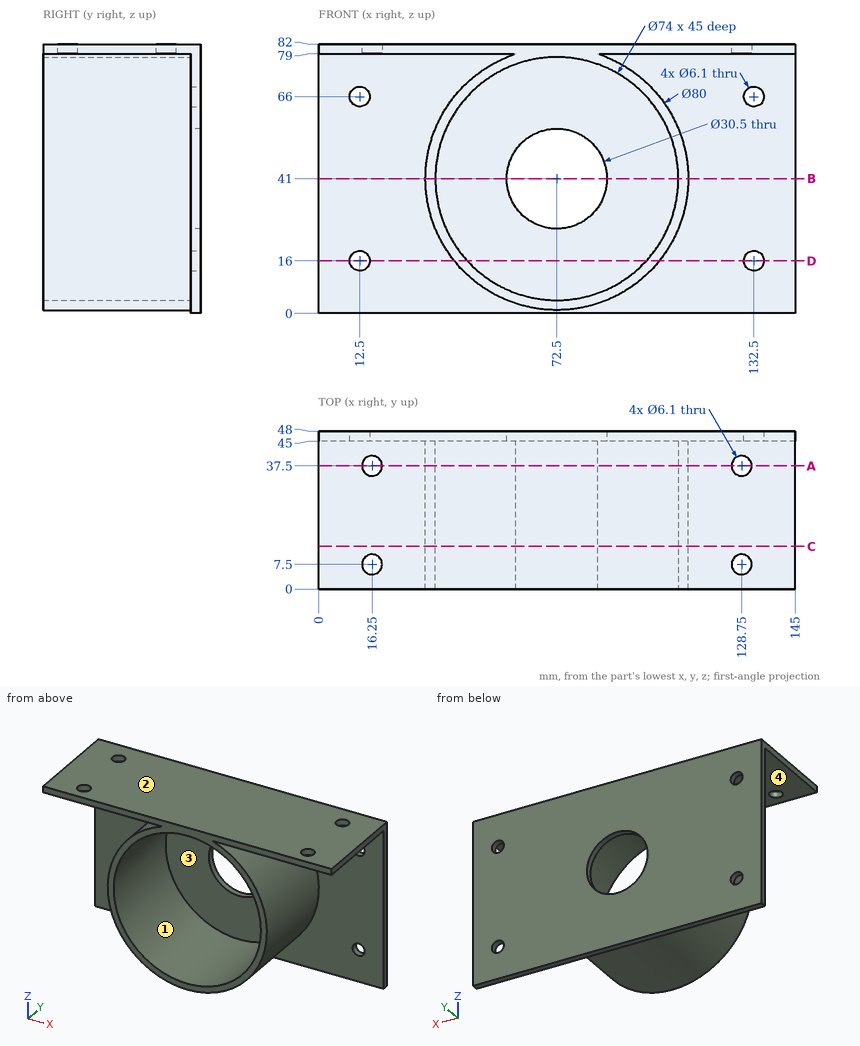
For this review, use the dimensioned drawing (mm, ordinates from the lowest corner) and the shaded views. A direction names the side the tool comes from. Coordinates: 2 decimals unless noted, no trailing zeros. Write each loop counter-clockwise with the first axis right and the second up, starting at its lowest first coordinate (ties: lowest second). Pieces come first, ordered by that corner, then holes. Notation, with made-up numbers: (-5.5, 50) -> (36.5, 50) arc R27 ccw to (36.5, 85) -> close; hole circle Ø6 at (-17, -36). An arc over 180 degrees is marked (long way). Put each result on its own line as item: value.
Q1. Take a section at D-D, the plane z = 16. State the section outline as (x, y) points, then the cut area to 3 significant figures.
From the geometry:
outline: (0, 45) -> (9.45, 45) -> (9.45, 48) -> (0, 48) -> close; (15.55, 45) -> (41.28, 45) -> (41.28, 0) -> (45.22, 0) -> (45.22, 45) -> (99.78, 45) -> (99.78, 0) -> (103.72, 0) -> (103.72, 45) -> (129.45, 45) -> (129.45, 48) -> (15.55, 48) -> close; (135.55, 45) -> (145, 45) -> (145, 48) -> (135.55, 48) -> close
area: 754 mm2
Q2. Tool access review of the marked faces 1 and 2: name each direction out of +Z, -Z, +X, -X, +Y, -Y from which nothing blocks a thin tool from reaching the whole face with its end or side.
From the geometry:
face 1: -Y
face 2: +Z, +X, -X, +Y, -Y
Q3. Clearance check with flat-ended pins moving along their axes: pin 1 Ø8 at (x, z) = (12.5, 66) entering from -Y; pin 2 Ø1 at (x, y) = (105.5, 36.5) entering from -Z; pin 3 Ø1 at (y, z) = (24.5, 35) entering from -X. State where each tip first meets the part, or that it passes through.
From the geometry:
pin 1: stops at y = 45
pin 2: stops at z = 17.68
pin 3: stops at x = 32.88
Q4. Take a section at C-C, the plane y = 13. State the section outline as (x, z) points, then the cut area to 3 significant figures.
From the geometry:
outline: (0, 79) -> (60.01, 79) arc R40 ccw (long way) to (84.99, 79) -> (145, 79) -> (145, 82) -> (0, 82) -> close; hole circle Ø74 at (72.5, 41)
area: 1,130 mm2
Q5. Take a section at B-B, the plane z = 41. State the section outline as (x, y) points.
From the geometry:
outline: (0, 45) -> (32.5, 45) -> (32.5, 0) -> (35.5, 0) -> (35.5, 45) -> (57.25, 45) -> (57.25, 48) -> (0, 48) -> close; (87.75, 45) -> (109.5, 45) -> (109.5, 0) -> (112.5, 0) -> (112.5, 45) -> (145, 45) -> (145, 48) -> (87.75, 48) -> close
Q6. Wall thickness on L1, parallel to X at y = 45.7, z = 16; L2, parallel to Y at x = 16.25, z = 79.8; L3, parallel to X at y = 37, z = 80: over which ranges is each line inside the solid? List them lowest first.
From the geometry:
L1: x = 0 to 9.45, 15.55 to 129.45, 135.55 to 145
L2: y = 0 to 4.45, 10.55 to 34.45, 40.55 to 48
L3: x = 0 to 13.24, 19.26 to 125.74, 131.76 to 145
Q7. Take a section at A-A, the plane y = 37.5. State the section outline as (x, z) points, then the cut area to 3 significant figures.
From the geometry:
outline: (0, 79) -> (13.2, 79) -> (13.2, 82) -> (0, 82) -> close; (19.3, 79) -> (60.01, 79) arc R40 ccw (long way) to (84.99, 79) -> (125.7, 79) -> (125.7, 82) -> (19.3, 82) -> close; (131.8, 79) -> (145, 79) -> (145, 82) -> (131.8, 82) -> close; hole circle Ø74 at (72.5, 41)
area: 1,090 mm2
Q8. The part is to be moulded in two halves that separate along X. For the marked faces 3 and 4, say which applies: +X half, -X half, draft (parallel to the pull), parting line (faces both ways), or undercut.
From the geometry:
face 3: undercut
face 4: draft
